from build123d import *

# Parameters (mm, degrees)
F0_W     = 20
F0_H     = 5
F1_DEPTH = 500
F2_R     = 12.5
F3_DEPTH = 50


with BuildPart() as f1:
    # F0 (on Top) → F1 (new body)
    with BuildSketch(Plane.XY):
        with BuildLine():
            Line((-9.995486, -11.592771), (-9.995486, 27.50601))
            ThreePointArc((-9.995486, 27.50601), (-12.499174, 28.243273), (-14.995486, 29.005138))
            Line((-14.995486, 29.005138), (-14.995486, -16.592771))
            Line((-14.995486, -16.592771), (-9.995486, -16.592771))
            Line((-9.995486, -16.592771), (-9.995486, -11.592771))
        make_face()
        with Locations((0.004514, -14.092771)):
            Rectangle(F0_W, F0_H)
        with BuildLine():
            Line((15.004514, -16.592771), (15.004514, 21.573286))
            ThreePointArc((15.004514, 21.573286), (12.502153, 22.05284), (10.004514, 22.55641))
            Line((10.004514, 22.55641), (10.004514, -11.592771))
            Line((10.004514, -11.592771), (10.004514, -16.592771))
            Line((10.004514, -16.592771), (15.004514, -16.592771))
        make_face()
    extrude(amount=F1_DEPTH)

    # F2 (on face) → F3 (cut)
    with BuildSketch(Plane.YZ.offset(15.004514)):
        with Locations((2.490257, 475)):
            Circle(F2_R)
    extrude(amount=-F3_DEPTH, mode=Mode.SUBTRACT)


with BuildPart() as f4_1:
    # F4: instance of F1
    add(f1.part.mirror(Plane.YZ))


solid = f4_1.part
The listing builds one solid part. Answer for the finished solid, in the listing's coordinates (mm). A direction names the side the tool comes from. Give positions to 0.01 mm unless a question says otherwise; leave off trailing zeros. Loops run counter-clockwise (first coordinate to the right, second up) from the corner with the lowest first, then second, coordinate; pieces in that order, holes last. Notation, with made-up numbers: M 32,-14 L 36,-14 A24 ccw 36,3 Z; hole C 84,36 d7. An arc over 180 degrees is marked long. Answer as CSV lines item,"result".
Item 1: Straight lines are drawn through the part: line 1 along X through (y, z) = (19, 119.5); line 2 along Z through (x, y) = (12, 1); line 3 along Y through (x, z) = (-9.75, 364.5). For each, find the intervals that lie inside material, in ascending order. Write a range as [from, to].
Values follow:
line 1,"x = [-15, -10], [10, 15]"
line 2,"z = [0, 462.59], [487.41, 500]"
line 3,"y = [-16.59, -11.59]"
Item 2: The mould has two halves that part along X. Classify faces 1 (the flat face through (0, -16.593, 246)), 2 (the flat face through (0, -11.593, 246)), 3 (the flat face through (14.995, 7, 246)), 4 (the flat face through (-10.005, 6, 246)): released by +X, released by -X, zero draft, split by the parting line, or undercut.
Values follow:
face 1,"zero draft"
face 2,"undercut"
face 3,"released by +X"
face 4,"undercut"
Item 3: The part is cut by section C-C (y = 5.5). Give the vertices of the cut face in (x, z), and give its area (3 significant figures).
Values follow:
outline,"M -15,0 L -10,0 L -10,462.87 L -15,462.87 Z; M -15,487.13 L -10,487.13 L -10,500 L -15,500 Z; M 10,0 L 15,0 L 15,462.87 L 10,462.87 Z; M 10,487.13 L 15,487.13 L 15,500 L 10,500 Z"
area,"4,760 mm^2"
Item 4: The part is cut by section B-B (z = 179). Give the vertices of the cut face in (x, y).
Values follow:
outline,"M -15,-16.59 L 15,-16.59 L 15,29.01 A265.22 cw 10,27.51 L 10,-11.59 L -10,-11.59 L -10,22.56 A265.23 cw -15,21.57 Z"
Item 5: Which of the six approach directions +Z, -Z, +X, -X, +Y, -Y give full straight-line access (tool end or side, diameter ignored) to faces 5 (the cylindrical face through (-12.54, 8.26, 463.91)), 6 (the flat face through (9.995, 8, 246))?
Values follow:
face 5,"+X, -X"
face 6,"+Z, -Z, +Y"
Item 6: The part is cut by section D-D (x = -1.5). Give the vertices of the cut face in (y, z), and give its area (3 significant figures).
Values follow:
outline,"M -16.59,0 L -11.59,0 L -11.59,500 L -16.59,500 Z"
area,"2,500 mm^2"
Item 7: Given pin 1 Ø1.5 at (x, z) = (0.5, 268.5) entering from +Y, flat-ended and moving along its own axis, determine where the tip first touches the part or whether it passes through.
Values follow:
pin 1,"stops at y = -11.59"
Item 8: The part is cut by section A-A (z = 475). Give the vertices of the cut face in (x, y).
Values follow:
outline,"M -15,-16.59 L 15,-16.59 L 15,-10.01 L 10,-10.01 L 10,-11.59 L -10,-11.59 L -10,-10.01 L -15,-10.01 Z; M -15,14.99 L -10,14.99 L -10,22.56 A265.23 cw -15,21.57 Z; M 10,14.99 L 15,14.99 L 15,29.01 A265.22 cw 10,27.51 Z"
